Drawing for the job (mm, zero at the part's lowest x, y, z). Coordinates: 2 decimals unless noted, no trailing zeros. Write each loop counter-clockwise with the first axis right and the second up, starting at its lowest first coordinate (ties: lowest second). Pieces come first, ordered by that corner, then holes. Notation, with made-up numbers: M 60.25,58 L 109.25,58 A23 cw 109.25,76 Z; hole C 48,-25 d8. An arc over 180 degrees is marked long. Put each result on its own line as item: value. Start each with the question number.
Q1. Cut at D-D (z = 3.3). Write the cut outline in (x, y).
Q2. Drill centre lines: line 1 along Y through (x, z) = (10, 1.6); line 2 along X through (y, z) = (8.75, 3.4); line 3 along X through (y, z) = (8.75, 0.75). Where is each one in solid material? Low to high.
Q3. Drop flat-ended pins along their axis: pin 1 (1 mm diameter, centred on y = 12.5, z = 3, fed in from -X); pin 2 (3 mm diameter, centred on x = 10, y = 10, fed in from -Z); pin 3 (1 mm diameter, centred on y = 3.5, z = 1, fed in from +X); pin 4 (6 mm diameter, centred on x = 4, y = 4.5, fed in from -Z). Give the stop position or say it passes through.
Q4. Pull direction X, two halves, no side cores. Call the marked faces 1, 2 and 3: pulls with the +X half, pulls with the -X half, needs draft (parallel to the pull), parting line crosses it, or undercut.
Q5. Cut at C-C (z = 1.5). Write the cut outline in (x, y), then the cut area to 3 significant figures.
Q6. Cut at A-A (y = 10). Write the cut outline in (x, z), then the cut area to 3 significant figures.
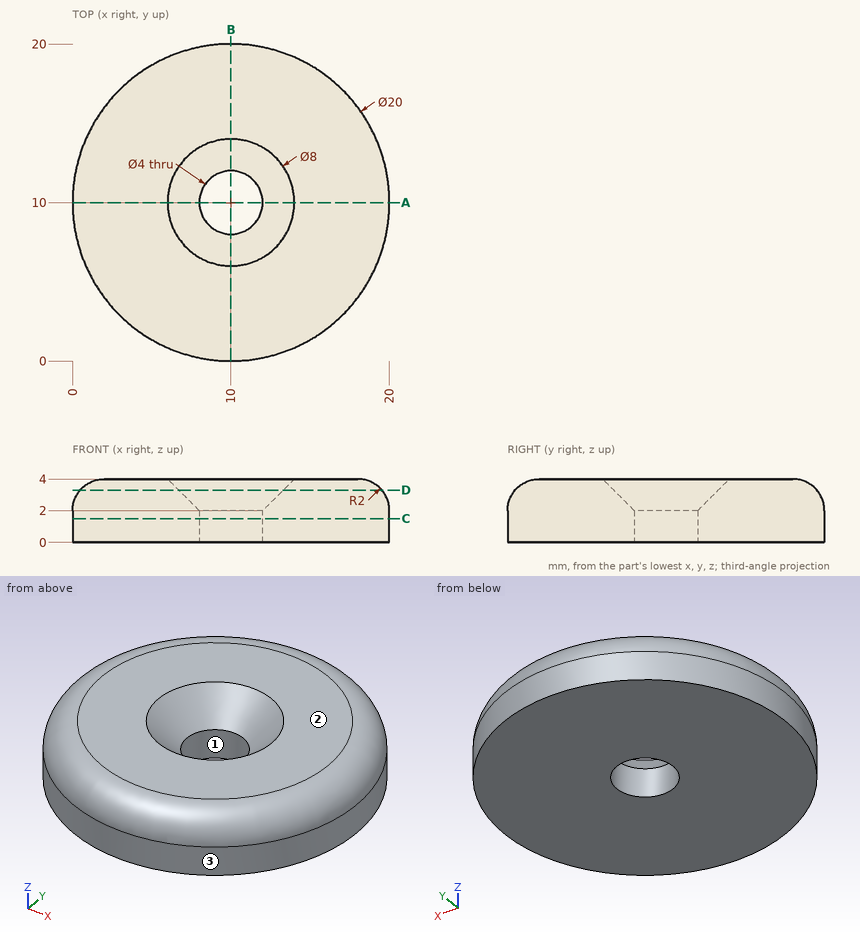
Computed values:
1. outline: C 10,10 d19.04; hole C 10,10 d6.6
2. line 1: 0 to 8, 12 to 20
2. line 2: 0.65 to 6.84, 13.16 to 19.35
2. line 3: 0.08 to 8.44, 11.56 to 19.92
3. pin 1: x = 0.34
3. pin 2: through
3. pin 3: x = 18
3. pin 4: z = 0
4. face 1: undercut
4. face 2: needs draft
4. face 3: parting line crosses it
5. outline: C 10,10 d20; hole C 10,10 d4
5. area: 302 mm2
6. outline: M 0,0 L 8,0 L 8,2 L 6,4 L 2,4 A2 ccw 0,2 Z; M 12,0 L 20,0 L 20,2 A2 ccw 18,4 L 14,4 L 12,2 Z
6. area: 58.3 mm2
